Geometry: final body of the model. Coordinates: model frame, mm. Face numbers are marked on the shaded views. A direction names the side the tool comes from. Give positions to 0.01 mm unless a question says otherwise; leave off trailing zeros. Write each loop counter-clockwise with the first axis right and the second up, starting at its lowest first coordinate (ties: lowest second). Pieces come first, ordered by that corner, then holes. Notation, with made-up numbers: M 26.5,83.5 L 39.5,83.5 A32 cw 39.5,116.5 Z; hole C 0,9.25 d1. An arc over 180 degrees is marked long. Use a Markdown table: item, result. Add a question column.
(1) Cut plane D-D (z = 16.5). Output: boundary loops of the cut face in (x, y), plus the area to 3 significant figures.
(2) Draft query along X for the marked faces 3, 4, 5 and 6. Return one class per face: released by +X, released by -X, zero draft, split by the parting line, or undercut.
(3) Cut plane C-C (y = -11). Output: boundary loops of the cut face in (x, z).
(4) Cut plane B-B (z = -16). Output: boundary loops of the cut face in (x, y).
(5) Material intervals for L1, parallel to Y at x = 19, z = -15.5; L2, parallel to X at y = 1.1, z = 0; L3, parallel to X at y = -9, z = -8.5, sorted ascending.
(6) Cut plane A-A (x = 0). Output: boundary loops of the cut face in (y, z).
(7) Pin query (flat end, axial travel): pin 1 Ø22 at (x, y) = (-1, -30) entering from +Z. Return the tip coordinate at first contact, or that it passes through.
(8) Reachability of the marked faces 1 and 2 from +Z, -Z, +X, -X, +Y, -Y: full face, straight path, thin tool, end or side. Return the list, or none.
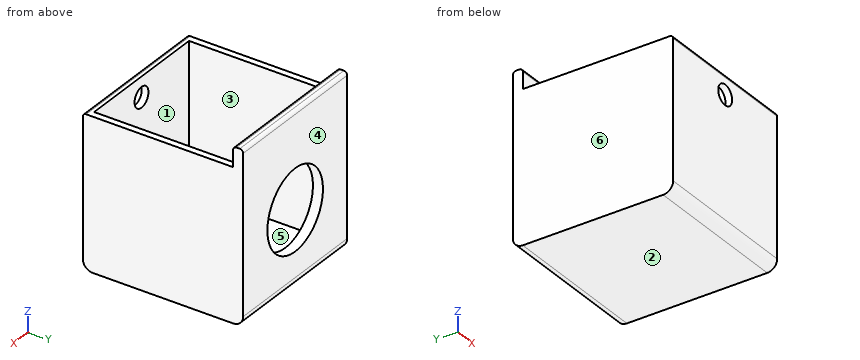
```python
from build123d import *

# Parameters (mm, degrees)
SKETCH_1_W          = 45
SKETCH_1_H          = 45
EXTRUDE_1_DEPTH     = 3
SKETCH_2_R          = 12
CUT_EXTRUDE_1_DEPTH = 3
SKETCH_3_W          = 2
SKETCH_3_H          = 45
EXTRUDE_3_DEPTH     = 45
SKETCH_4_R          = 12
CUT_EXTRUDE_2_DEPTH = 3
SKETCH_5_W          = 41
SKETCH_5_H          = 2
EXTRUDE_4_DEPTH     = 45
SKETCH_6_W          = 41
SKETCH_6_H          = 2
EXTRUDE_5_DEPTH     = 43
SKETCH_8_W          = 45
SKETCH_8_H          = 3
EXTRUDE_6_DEPTH     = 6
FILLET_3_R          = 1
FILLET_4_R          = 3
SKETCH_9_R          = 3
CUT_EXTRUDE_3_DEPTH = 2
FILLET_8_R          = 1


with BuildPart() as part:
    # Эскиз1 → Бобышка-Вытянуть1 (new body)
    with BuildSketch(Plane(origin=(0, 0, 0), x_dir=(1, 0, 0), z_dir=(0, 1, 0))):
        Rectangle(SKETCH_1_W, SKETCH_1_H)
    extrude_1 = extrude(amount=EXTRUDE_1_DEPTH)

    # Эскиз2 → Вырез-Вытянуть1 (cut)
    with BuildSketch(Plane(origin=(0, 3, 0), x_dir=(1, 0, 0), z_dir=(0, 1, 0))):
        Circle(SKETCH_2_R)
    extrude(amount=-CUT_EXTRUDE_1_DEPTH, mode=Mode.SUBTRACT)

    # Эскиз3 → Бобышка-Вытянуть3 (add)
    with BuildSketch(Plane.XZ):
        with Locations((-21.5, 0)):
            Rectangle(SKETCH_3_W, SKETCH_3_H)
    extrude_3 = extrude(amount=EXTRUDE_3_DEPTH)

    # Зеркальное отражение3: Бобышка-Вытянуть1, Бобышка-Вытянуть3 across plane
    add(extrude_1.mirror(Plane.ZY))
    add(extrude_3.mirror(Plane.ZY))

    # Эскиз4 → Вырез-Вытянуть2 (cut)
    with BuildSketch(Plane(origin=(0, 3, 0), x_dir=(1, 0, 0), z_dir=(0, 1, 0))):
        Circle(SKETCH_4_R)
    extrude(amount=-CUT_EXTRUDE_2_DEPTH, mode=Mode.SUBTRACT)

    # Эскиз5 → Бобышка-Вытянуть4 (add)
    with BuildSketch(Plane.XZ):
        with Locations((0, -21.5)):
            Rectangle(SKETCH_5_W, SKETCH_5_H)
    extrude(amount=EXTRUDE_4_DEPTH)

    # Эскиз6 → Бобышка-Вытянуть5 (add)
    with BuildSketch(Plane.XY.offset(-20.5)):
        with Locations((0, -44)):
            Rectangle(SKETCH_6_W, SKETCH_6_H)
    extrude(amount=EXTRUDE_5_DEPTH)

    # Эскиз8 → Бобышка-Вытянуть6 (add)
    with BuildSketch(Plane.XY.offset(22.5)):
        with Locations((0, 1.5)):
            Rectangle(SKETCH_8_W, SKETCH_8_H)
    extrude(amount=EXTRUDE_6_DEPTH)

    # Скругление3
    fillet_3_edges = [part.edges().sort_by_distance(p)[0] for p in [
        (0, 0, 28.5),
        (0, 3, 28.5),
    ]]
    fillet(fillet_3_edges, radius=FILLET_3_R)

    # Скругление4
    fillet_4_edges = [part.edges().sort_by_distance(p)[0] for p in [
        (0, -45, -22.5),
        (0, 3, -22.5),
    ]]
    fillet(fillet_4_edges, radius=FILLET_4_R)

    # Эскиз9 → Вырез-Вытянуть3 (cut)
    with BuildSketch(Plane.XZ.offset(45)):
        with Locations((0, 16.5)):
            Circle(SKETCH_9_R)
    extrude(amount=-CUT_EXTRUDE_3_DEPTH, mode=Mode.SUBTRACT)

    # Скругление8
    fillet_8_edges = [part.edges().sort_by_distance(p)[0] for p in [
        (0, -45, 22.5),
    ]]
    fillet(fillet_8_edges, radius=FILLET_8_R)


solid = part.part
```
Answer list:
| question | item | result |
|---|---|---|
| 1 | outline | M -22.5,-45 L -3,-45 L -3,-43 L -20.5,-43 L -20.5,0 L 20.5,0 L 20.5,-43 L 3,-43 L 3,-45 L 22.5,-45 L 22.5,3 L -22.5,3 Z |
| 1 | area | 385 mm² |
| 2 | face 3 | undercut |
| 2 | face 4 | zero draft |
| 2 | face 5 | undercut |
| 2 | face 6 | released by -X |
| 3 | outline | M -22.5,-22.5 L 22.5,-22.5 L 22.5,22.5 L 20.5,22.5 L 20.5,-20.5 L -20.5,-20.5 L -20.5,22.5 L -22.5,22.5 Z |
| 4 | outline | M -22.5,-45 L 22.5,-45 L 22.5,3 L -22.5,3 Z; hole M -20.5,-43 L 20.5,-43 L 20.5,0 L -20.5,0 Z |
| 5 | L1 | -45 to -43, 0 to 3 |
| 5 | L2 | -22.5 to -12, 12 to 22.5 |
| 5 | L3 | -22.5 to -20.5, 20.5 to 22.5 |
| 6 | outline | M -45,-19.5 A3 ccw -42,-22.5 L 0,-22.5 A3 ccw 3,-19.5 L 3,-12 L 0,-12 L 0,-20.5 L -43,-20.5 L -43,13.5 L -45,13.5 Z; M -45,19.5 L -43,19.5 L -43,22.5 L -44,22.5 A1 ccw -45,21.5 Z; M 0,12 L 3,12 L 3,27.5 A1 ccw 2,28.5 L 1,28.5 A1 ccw 0,27.5 Z |
| 7 | pin 1 | z = -20.5 |
| 8 | face 1 | +Z |
| 8 | face 2 | -Z, +X, -X, +Y, -Y |
